Verification items for the finished model (mm, model axes). Round coordinates to 2 decimals unless told otherwise and drop trailing zeros. Write each loop counter-clockwise with the first axis right and the second up, starting at its lowest first coordinate (ties: lowest second). Pieces come first, ordered by that corner, then holes. Notation, with made-up numbers: (4, 15.25) -> (41, 15.25) arc R26 cw to (41, 45.25) -> close; hole circle Ø10 at (80, -21.75). An arc over 180 degrees is marked (long way). Answer as a JSON object with one key per item and string values. Group by question number.
(1) Sectioned sample at B-B on z = 0.5. Record the cut outline in (x, y), and give its area (3 significant figures).
(2) Scan lines: L1, parallel to Y at x = 4, z = 3.4; L2, parallel to Y at x = 6, z = 0.9; L3, parallel to X at y = 4, z = 2.5. Record each from-to range of solid material in increasing order. Write a range as from..to.
(3) Sectioned sample at D-D on y = 1. Record the cut outline in (x, z).
(4) Gauge pin test, flat end, axial feed: pin 1 Ø4 at (x, y) = (4.11, 5) entering from -Z. Record the tip position at first contact, or that the pin passes through.
(5) Sectioned sample at A-A on z = 2.5. Record the cut outline in (x, y).
(6) Draft check along Y on faces 1 (the face through (15, 5, 0)), 2 (the face through (3.74, 3.34, 2.74)), 3 (the face through (10, 10, 2)). Enter one of: released by +Y, released by -Y, zero draft, split by the parting line, or undercut.
(7) Sectioned sample at C-C on x = 25.5. Record the cut outline in (y, z).
```python
from build123d import *

# Parameters (mm, degrees)
EXTRUSION1_DEPTH                               = 4
FRAISAGE_POUR_VIS_T_TE_FRAIS_E_M31_D           = 3.4
FRAISAGE_POUR_VIS_T_TE_FRAIS_E_M31_CSINK_D     = 6.3
FRAISAGE_POUR_VIS_T_TE_FRAIS_E_M31_CSINK_ANGLE = 90


with BuildPart() as part:
    # Esquisse1 → Extrusion1 (new body)
    with BuildSketch(Plane.XY):
        Polygon((0, 0), (0, 10), (21.146637523, 10), (30, 0), align=None)
    extrude(amount=EXTRUSION1_DEPTH)

    # Fraisage pour vis à tête fraisée M31 (through all)
    with Locations(Plane(origin=(4.111822058, 5, 0), x_dir=(-1, 0, 0), z_dir=(0, 0, -1))):
        with Locations((0, 0)):
            CounterSinkHole(FRAISAGE_POUR_VIS_T_TE_FRAIS_E_M31_D / 2, FRAISAGE_POUR_VIS_T_TE_FRAIS_E_M31_CSINK_D / 2, counter_sink_angle=FRAISAGE_POUR_VIS_T_TE_FRAIS_E_M31_CSINK_ANGLE)


solid = part.part
```
Computed values:
{
 "1": {"outline": "(0, 0) -> (30, 0) -> (21.15, 10) -> (0, 10) -> close; hole circle Ø5.3 at (4.11, 5)", "area": "234 mm2"},
 "2": {"L1": "0..3.3, 6.7..10", "L2": "0..3.78, 6.22..10", "L3": "0..2.74, 5.49..26.46"},
 "3": {"outline": "(0, 0) -> (29.11, 0) -> (29.11, 4) -> (0, 4) -> close"},
 "4": {"pin 1": "z = 1.15"},
 "5": {"outline": "(0, 0) -> (30, 0) -> (21.15, 10) -> (0, 10) -> close; hole circle Ø3.4 at (4.11, 5)"},
 "6": {"face 1": "zero draft", "face 2": "undercut", "face 3": "released by +Y"},
 "7": {"outline": "(0, 0) -> (5.08, 0) -> (5.08, 4) -> (0, 4) -> close"}
}
